```python
from build123d import *

# Parameters (mm, degrees)
SKETCH1_R           = 1.6
BOSS_EXTRUDE1_DEPTH = 8
CHAMFER1_SIZE       = 1


with BuildPart() as part:
    # Sketch1 → Boss-Extrude1 (new body)
    with BuildSketch(Plane.XY):
        with BuildLine():
            Line((-0.5, 3), (30.5, 3))
            ThreePointArc((30.5, 3), (32.267766953, 2.267766953), (33, 0.5))
            Line((33, 0.5), (33, -0.5))
            ThreePointArc((33, -0.5), (32.267766953, -2.267766953), (30.5, -3))
            Line((30.5, -3), (-0.5, -3))
            ThreePointArc((-0.5, -3), (-2.267766953, -2.267766953), (-3, -0.5))
            Line((-3, -0.5), (-3, 0.5))
            ThreePointArc((-3, 0.5), (-2.267766953, 2.267766953), (-0.5, 3))
        make_face()
        Circle(SKETCH1_R, mode=Mode.SUBTRACT)
        with Locations((7.5, 0)):
            Circle(SKETCH1_R, mode=Mode.SUBTRACT)
        with Locations((15, 0)):
            Circle(SKETCH1_R, mode=Mode.SUBTRACT)
        with Locations((22.5, 0)):
            Circle(SKETCH1_R, mode=Mode.SUBTRACT)
        with Locations((30, 0)):
            Circle(SKETCH1_R, mode=Mode.SUBTRACT)
    extrude(amount=BOSS_EXTRUDE1_DEPTH)

    # Chamfer1
    chamfer1_edges = [part.edges().sort_by_distance(p)[0] for p in [
        (-1.6, 0, 0),
        (-1.6, 0, 8),
        (5.9, 0, 0),
        (5.9, 0, 8),
        (13.4, 0, 0),
        (13.4, 0, 8),
        (20.9, 0, 0),
        (20.9, 0, 8),
        (28.4, 0, 0),
        (28.4, 0, 8),
    ]]
    chamfer(chamfer1_edges, length=CHAMFER1_SIZE)


solid = part.part
```
CAD build for the part. Positions are in the model's coordinates, mm. Round coordinates to 2 decimals unless told otherwise and drop trailing zeros. Order: outer loops, then holes, each group sorted by start corner. A loop starts at its lowest first (then second) coordinate and runs counter-clockwise, first axis right, second up.
Item 1: Mould opens along X. For faces 1 (the face through (15, -3, 4)), 2 (the face through (-3, 0, 4)), 3 (the face through (32.248, 2.287, 3.944)), 4 (the face through (28.4, 0.07, 3.96)) say: pulls with the +X half, pulls with the -X half, needs draft (parallel to the pull), parting line crosses it, or undercut.
Item 2: Saw through at B-B on z = 0.5. Write the cut outline in (x, y), then the cut area to 3 significant figures.
Item 3: Probe line 1 along Y through (x, z) = (15, 5.5); line 2 along X through (y, z) = (0.7, 7.75); line 3 along X through (y, z) = (-0.75, 3.25). List the from-to ranges inside material, lowest first.
Item 4: Pin check, flat tip, straight feed: pin 1 (3.5 mm diameter, centred on x = 0, y = 0, fed in from -Z). Stop position of the tip, or through.
Item 5: Saw through at A-A on x = 30. Write the cut outline in (y, z).
Item 6: Saw through at C-C on y = 0. State how many separate pieces and enclosed holes the cut face has, then the cut area to 3 significant figures.
Item 7: Saw through at D-D on z = 5. Write the cut outline in (x, y).
Reported:
1. face 1: needs draft
1. face 2: pulls with the -X half
1. face 3: pulls with the +X half
1. face 4: undercut
2. outline: (-3, -0.5) arc R2.5 ccw to (-0.5, -3) - (30.5, -3) arc R2.5 ccw to (33, -0.5) - (33, 0.5) arc R2.5 ccw to (30.5, 3) - (-0.5, 3) arc R2.5 ccw to (-3, 0.5) - close; hole circle Ø4.2 at (0, 0); hole circle Ø4.2 at (7.5, 0); hole circle Ø4.2 at (15, 0); hole circle Ø4.2 at (22.5, 0); hole circle Ø4.2 at (30, 0)
2. area: 141 mm2
3. line 1: y = -3 to -1.6, 1.6 to 3
3. line 2: x = -2.99 to -2.24, 2.24 to 5.26, 9.74 to 12.76, 17.24 to 20.26, 24.74 to 27.76, 32.24 to 32.99
3. line 3: x = -2.99 to -1.41, 1.41 to 6.09, 8.91 to 13.59, 16.41 to 21.09, 23.91 to 28.59, 31.41 to 32.99
4. pin 1: stops at z = 0.85
5. outline: (-3, 0) - (-2.6, 0) - (-1.6, 1) - (-1.6, 7) - (-2.6, 8) - (-3, 8) - close; (1.6, 1) - (2.6, 0) - (3, 0) - (3, 8) - (2.6, 8) - (1.6, 7) - close
6. separate pieces: 6
6. enclosed holes: 0
6. area: 150 mm2
7. outline: (-3, -0.5) arc R2.5 ccw to (-0.5, -3) - (30.5, -3) arc R2.5 ccw to (33, -0.5) - (33, 0.5) arc R2.5 ccw to (30.5, 3) - (-0.5, 3) arc R2.5 ccw to (-3, 0.5) - close; hole circle Ø3.2 at (0, 0); hole circle Ø3.2 at (7.5, 0); hole circle Ø3.2 at (15, 0); hole circle Ø3.2 at (22.5, 0); hole circle Ø3.2 at (30, 0)
